Source: CAD feature listing. Evaluate the final solid. Frame: model axes, mm. A direction names the side the tool comes from. Coordinates: 2 decimals unless noted, no trailing zeros. Order: outer loops, then holes, each group sorted by start corner. A loop starts at its lowest first (then second) coordinate and runs counter-clockwise, first axis right, second up. Notation, with made-up numbers: (42.25, 64) -> (100.25, 64) arc R22 ccw to (100.25, 95) -> close; hole circle Ø9 at (-21, -33.5). An arc over 180 degrees is marked (long way). Put each result on its own line as item: value.
from build123d import *

# Parameters (mm, degrees)
SKETCH1_W               = 518.953439809
SKETCH1_H               = 518.249184403
SKETCH1_W_2             = 455.6
BOSS_EXTRUDE3_DEPTH     = 80
SKETCH2_W               = 101.131848524
SKETCH2_H               = 50
SKETCH2_W_2             = 87.153604081
BOSS_EXTRUDE4_DEPTH     = 160
FILLET1_R               = 20
CUT_EXTRUDE3_DEPTH      = 1373.160931607
CUT_EXTRUDE3_DEPTH_BACK = 10
SKETCH5_R               = 20
CUT_EXTRUDE4_DEPTH      = 1382.534741242
CUT_EXTRUDE4_DEPTH_BACK = 1382.534741242
SKETCH3_R               = 20
CUT_EXTRUDE5_DEPTH      = 1382.534741304
CUT_EXTRUDE5_DEPTH_BACK = 1382.534741304
SKETCH4_R               = 20
SKETCH6_W               = 101.131848524
SKETCH6_H               = 50
BOSS_EXTRUDE5_DEPTH     = 60
CUT_EXTRUDE6_DEPTH      = 1394.211484888
CUT_EXTRUDE6_DEPTH_BACK = 1394.211484888
SKETCH7_R               = 20
SKETCH8_W               = 87.153604081
SKETCH8_H               = 50
BOSS_EXTRUDE6_DEPTH     = 60
CUT_EXTRUDE7_DEPTH      = 1394.211484888
CUT_EXTRUDE7_DEPTH_BACK = 1394.211484888
SKETCH9_R               = 20


with BuildPart() as part:
    # Sketch1 → Boss-Extrude3 (new body)
    with BuildSketch(Plane(origin=(0, 0, 0), x_dir=(1, 0, 0), z_dir=(0, 1, 0))):
        Polygon((-121.456854781, 21.240444949), (1211.943145219, 21.240444949), (1211.943145219, -50.701004169), (1211.943145219, -568.950188572), (1211.943145219, -597.008739454), (-121.456854781, -597.008739454), (-121.456854781, -547.008739454), (87.38970541, -547.008739454), (87.38970541, -28.759555051), (-121.456854781, -28.759555051), align=None)
        with Locations((396.866425315, -287.884147253)):
            Rectangle(SKETCH1_W, SKETCH1_H, mode=Mode.SUBTRACT)
        with Locations((934.143145219, -287.884147253)):
            Rectangle(SKETCH1_W_2, SKETCH1_H, mode=Mode.SUBTRACT)
    extrude(amount=BOSS_EXTRUDE3_DEPTH)

    # Sketch2 → Boss-Extrude4 (add)
    with BuildSketch(Plane(origin=(0, 80, 0), x_dir=(1, 0, 0), z_dir=(0, 1, 0))):
        with Locations((605.777220957, -3.759555051)):
            Rectangle(SKETCH2_W, SKETCH2_H)
        with Locations((1168.366343179, -3.759555051)):
            Rectangle(SKETCH2_W_2, SKETCH2_H)
        with Locations((605.777220957, -572.008739454)):
            Rectangle(SKETCH2_W, SKETCH2_H)
        with Locations((1168.366343179, -572.008739454)):
            Rectangle(SKETCH2_W_2, SKETCH2_H)
    extrude(amount=BOSS_EXTRUDE4_DEPTH)

    # Fillet1
    fillet1_edges = [part.edges().sort_by_distance(p)[0] for p in [
        (656.343145219, 240, 572.008739454),
        (605.777220957, 240, 547.008739454),
        (555.211296695, 240, 572.008739454),
        (605.777220957, 240, 597.008739454),
        (1124.789541138, 240, 3.759555051),
        (1168.366343178, 240, 28.759555051),
        (1211.943145219, 240, 3.759555051),
        (1168.366343178, 240, -21.240444949),
        (1124.789541138, 240, 572.008739454),
        (1168.366343178, 240, 597.008739454),
        (1211.943145219, 240, 572.008739454),
        (1168.366343178, 240, 547.008739454),
        (555.211296695, 240, 3.759555051),
        (605.777220957, 240, 28.759555051),
        (656.343145219, 240, 3.759555051),
        (605.777220957, 240, -21.240444949),
    ]]
    fillet(fillet1_edges, radius=FILLET1_R)

    # Sketch5 → Cut-Extrude3 (cut, two sides: drawn at the far end of the back side and taken through both)
    with BuildSketch(Plane(origin=(0, 0, 0), x_dir=(-1, 0, 0), z_dir=(0, -1, 0)).offset(-CUT_EXTRUDE3_DEPTH_BACK)):
        with Locations(Location((-1187.046867592, -287.884147253, 0), (0, 0, 270))):
            Circle(SKETCH5_R)
    extrude(amount=CUT_EXTRUDE3_DEPTH + CUT_EXTRUDE3_DEPTH_BACK, mode=Mode.SUBTRACT)

    # Sketch3 → Cut-Extrude4 (cut, two sides: drawn at the far end of the back side and taken through both)
    with BuildSketch(Plane(origin=(0, 0, -21.240444949), x_dir=(-1, 0, 0), z_dir=(0, 0, -1)).offset(-CUT_EXTRUDE4_DEPTH_BACK)):
        with Locations(Location((-604.119324359, 215.055032995, 0), (0, 0, 14.314743265))):
            Circle(SKETCH3_R)
    extrude(amount=CUT_EXTRUDE4_DEPTH + CUT_EXTRUDE4_DEPTH_BACK, mode=Mode.SUBTRACT)

    # Sketch4 → Cut-Extrude5 (cut, two sides: drawn at the far end of the back side and taken through both)
    with BuildSketch(Plane(origin=(0, 0, -21.240444949), x_dir=(-1, 0, 0), z_dir=(0, 0, -1)).offset(-CUT_EXTRUDE5_DEPTH_BACK)):
        with Locations(Location((-1171.400402377, 215.184793276, 0), (0, 0, 13.931420355))):
            Circle(SKETCH4_R)
    extrude(amount=CUT_EXTRUDE5_DEPTH + CUT_EXTRUDE5_DEPTH_BACK, mode=Mode.SUBTRACT)

    # Sketch6 → Boss-Extrude5 (add)
    with BuildSketch(Plane(origin=(0, 240, 0), x_dir=(1, 0, 0), z_dir=(0, 1, 0))):
        with Locations((605.777220957, -3.759555051)):
            Rectangle(SKETCH6_W, SKETCH6_H)
        with Locations((605.777220957, -572.008739454)):
            Rectangle(SKETCH6_W, SKETCH6_H)
    extrude(amount=BOSS_EXTRUDE5_DEPTH)

    # Sketch7 → Cut-Extrude6 (cut, two sides: drawn at the far end of the back side and taken through both)
    with BuildSketch(Plane.XY.offset(597.008739454).offset(-CUT_EXTRUDE6_DEPTH_BACK)):
        with Locations((604.119324359, 272.419198887)):
            Circle(SKETCH7_R)
    extrude(amount=CUT_EXTRUDE6_DEPTH + CUT_EXTRUDE6_DEPTH_BACK, mode=Mode.SUBTRACT)

    # Sketch8 → Boss-Extrude6 (add)
    with BuildSketch(Plane(origin=(0, 240, 0), x_dir=(1, 0, 0), z_dir=(0, 1, 0))):
        with Locations((1168.366343179, -572.008739454)):
            Rectangle(SKETCH8_W, SKETCH8_H)
        with Locations((1168.366343179, -3.759555051)):
            Rectangle(SKETCH8_W, SKETCH8_H)
    extrude(amount=BOSS_EXTRUDE6_DEPTH)

    # Sketch9 → Cut-Extrude7 (cut, two sides: drawn at the far end of the back side and taken through both)
    with BuildSketch(Plane.XY.offset(597.008739454).offset(-CUT_EXTRUDE7_DEPTH_BACK)):
        with Locations((1168.366343178, 271.00396048)):
            Circle(SKETCH9_R)
    extrude(amount=CUT_EXTRUDE7_DEPTH + CUT_EXTRUDE7_DEPTH_BACK, mode=Mode.SUBTRACT)


solid = part.part
1. First-contact query: pin 1 (25 mm diameter, centred on y = 149.5, z = 10.5, fed in from -X); pin 2 (4 mm diameter, centred on x = 579, y = 231.5, fed in from -Z); pin 3 (25 mm diameter, centred on x = 1192, z = 280.5, fed in from +Y). Flat tips, straight axial feed; report the tip coordinate or a pass-through.
Numbers:
pin 1: stops at x = 555.21
pin 2: stops at z = -18.84
pin 3: stops at y = 80
2. Cut plane D-D on y = 50.5. Output: boundary loops of the cut face in (x, z), plus the area to 3 significant figures.
Numbers:
outline: (-121.46, -21.24) -> (1211.94, -21.24) -> (1211.94, 597.01) -> (-121.46, 597.01) -> (-121.46, 547.01) -> (87.39, 547.01) -> (87.39, 28.76) -> (-121.46, 28.76) -> close; hole (137.39, 28.76) -> (656.34, 28.76) -> (656.34, 547.01) -> (137.39, 547.01) -> close; hole (706.34, 28.76) -> (1161.94, 28.76) -> (1161.94, 547.01) -> (706.34, 547.01) -> close
area: 211,000 mm2
3. Cut plane B-B on y = 107. Output: boundary loops of the cut face in (x, z), plus the area to 3 significant figures.
Numbers:
outline: (555.21, -21.24) -> (656.34, -21.24) -> (656.34, 28.76) -> (555.21, 28.76) -> close; (555.21, 547.01) -> (656.34, 547.01) -> (656.34, 597.01) -> (555.21, 597.01) -> close; (1124.79, -21.24) -> (1211.94, -21.24) -> (1211.94, 28.76) -> (1124.79, 28.76) -> close; (1124.79, 547.01) -> (1211.94, 547.01) -> (1211.94, 597.01) -> (1124.79, 597.01) -> close
area: 18,800 mm2
4. Pull-direction query (Y, two-part tool) for faces 5 (the flat face through (656.343, 149, 4)), 6 (the flat face through (605, 300, 3)), 7 (the cylindrical face through (1170.91, 195.19, 4.11)), 8 (the cylindrical face through (603.493, 195.065, 572.359)); classes: pulls with the +Y half, pulls with the -Y half, needs draft (parallel to the pull), parting line crosses it, or undercut.
Numbers:
face 5: needs draft
face 6: pulls with the +Y half
face 7: undercut
face 8: undercut
5. Cut plane C-C on x = 318.5. Output: boundary loops of the cut face in (y, z).
Numbers:
outline: (0, -21.24) -> (80, -21.24) -> (80, 28.76) -> (0, 28.76) -> close; (0, 547.01) -> (80, 547.01) -> (80, 597.01) -> (0, 597.01) -> close
6. Ray query, line 1 along X through (y, z) = (48.5, 296); line 2 along Z through (x, y) = (587, 134); line 3 along Y through (x, z) = (129, 85.5). Return the intervals inside material, ascending.
Numbers:
line 1: x = 87.39 to 137.39, 656.34 to 706.34, 1161.94 to 1211.94
line 2: z = -21.24 to 28.76, 547.01 to 597.01
line 3: y = 0 to 80
7. Cut plane A-A on z = 147. Output: boundary loops of the cut face in (x, y).
Numbers:
outline: (87.39, 0) -> (137.39, 0) -> (137.39, 80) -> (87.39, 80) -> close; (656.34, 0) -> (706.34, 0) -> (706.34, 80) -> (656.34, 80) -> close; (1161.94, 0) -> (1211.94, 0) -> (1211.94, 80) -> (1161.94, 80) -> close
8. Set-up query: faces 1 (the flat face through (616, 256, 547.009)), 2 (the flat face through (555.211, 149, 4)), 3 (the flat face through (656.343, 149, 572)), 4 (the flat face through (87.39, 39, 292)). Return all of +Z, -Z, +X, -X, +Y, -Y with unobstructed straight access to the full face (end or side cutting, diameter ignored); none if empty.
Numbers:
face 1: +X, -X, +Y, -Y
face 2: +Z, -Z, -X, +Y
face 3: +Z, -Z, +Y
face 4: -X, +Y, -Y
